Source: three-view drawing plus pictorial views. Frame: mm from the lowest corner of the part. A direction names the side the tool comes from. Give positions to 0.01 mm unless a question says otherwise; leave off trailing zeros. Order: outer loops, then holes, each group sorted by start corner. A loop starts at its lowest first (then second) coordinate and runs counter-clockwise, first axis right, second up. Notation, with made-up numbers: (62.25, 68.25) -> (72.25, 68.25) arc R30 ccw to (72.25, 102.25) -> close; hole circle Ø10 at (-9, -15.5). An arc over 180 degrees is marked (long way). Answer in a Markdown table with one row per item. Add a question column.
Q1. Set-up query: the marked faces 1, 2 and 3. Return all of +Z, -Z, +X, -X, +Y, -Y with unobstructed straight access to the full face (end or side cutting, diameter ignored); none if empty.
Q2. Cut plane C-C on x = 12. Return the cut outline in (y, z) (1 decimal).
Q3. Line query: line 1 along Z through (x, y) = (3, 85) (1 decimal); line 2 along Y through (x, z) = (49, 24); line 3 along Z through (x, y) = (48.5, 91.5) (1 decimal). Output: solid intervals per line, ascending. Write a range as from..to.
Q4. Contact query for flat-ended pins moving along their axis: P1, Ø6.5, axis at y = 52.5, z = 12, coming from the -X side (3 decimals); P2, Ø10.5, axis at y = 63, z = 13.5, coming from the +X side; P3, Ø3, axis at x = 20.5, y = 59.5, coming from the +Z side (3 decimals). Output: stop coordinate, or through.
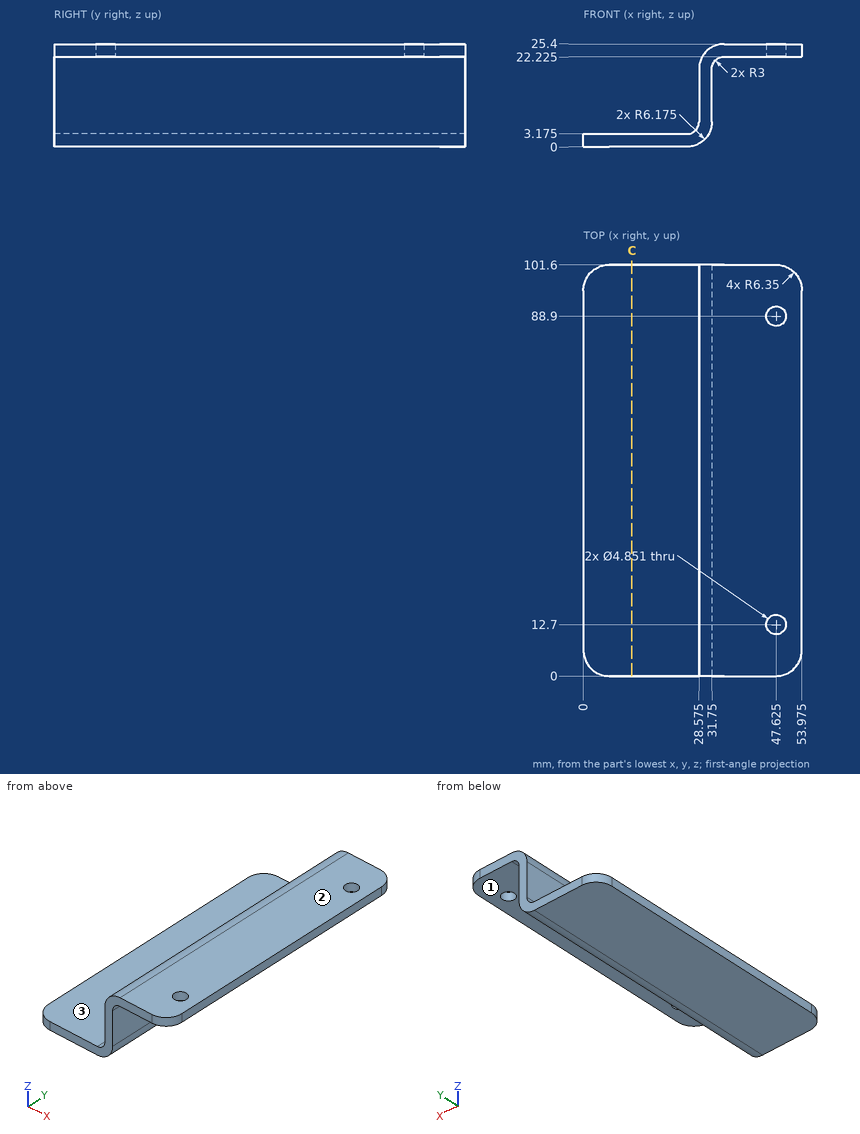
Completed:
| question | item | result |
|---|---|---|
| 1 | face 1 | -Z, +X, +Y, -Y |
| 1 | face 2 | +Z, +X, -X, +Y, -Y |
| 1 | face 3 | +Z, -X, +Y, -Y |
| 2 | outline | (0, 0) -> (101.6, 0) -> (101.6, 3.2) -> (0, 3.2) -> close |
| 3 | line 1 | z = 0..3.2 |
| 3 | line 2 | y = 0.15..10.7, 14.7..86.9, 90.9..101.45 |
| 3 | line 3 | z = 22.2..25.4 |
| 4 | P1 | stops at x = 28.575 |
| 4 | P2 | stops at x = 31.75 |
| 4 | P3 | stops at z = 3.175 |
